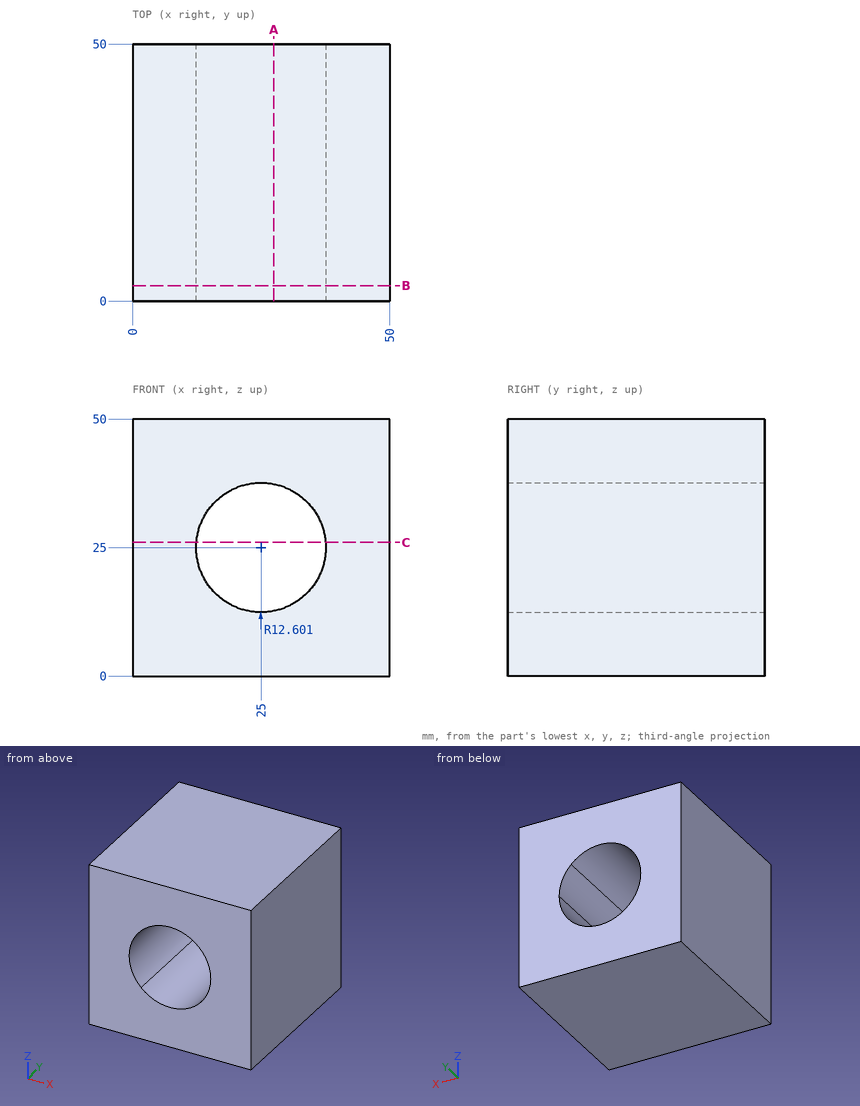
Print and shaded views of the part. All mm, measured from the part's lowest x, y and z. Round coordinates to 2 decimals unless told otherwise and drop trailing zeros. Write each loop counter-clockwise with the first axis right and the second up, starting at its lowest first coordinate (ties: lowest second). Pieces come first, ordered by that corner, then holes. Notation, with made-up numbers: (45.5, 68.5) -> (69.5, 68.5) arc R28 ccw to (69.5, 97.5) -> close; hole circle Ø1 at (28, -9.75). An arc over 180 degrees is marked (long way). Return JSON: item names as keys, results as strings. Group by question number.
Q1. Probe L1, parallel to Z at x = 30, y = 38 (1 decimal); L2, parallel to Z at x = 26, y = 14.5; L3, parallel to X at y = 19, z = 19.5. List the from-to ranges inside material, lowest first. Write a range as [from, to].
Q2. Saw through at B-B on y = 3. Write the cut outline in (x, z).
Q3. Saw through at C-C on z = 26. Write the cut outline in (x, y).
Q4. Saw through at A-A on x = 27.5. Write the cut outline in (y, z).
Answer:
{
 "1": {"L1": "[0, 13.4], [36.6, 50]", "L2": "[0, 12.44], [37.56, 50]", "L3": "[0, 13.66], [36.34, 50]"},
 "2": {"outline": "(0, 0) -> (50, 0) -> (50, 50) -> (0, 50) -> close; hole (16.09, 16.09) arc R12.6 ccw to (33.91, 16.09) arc R12.6 ccw to (37.6, 25) arc R12.6 ccw to (33.91, 33.91) arc R12.6 ccw to (16.09, 33.91) arc R12.6 ccw to start"},
 "3": {"outline": "(0, 0) -> (12.44, 0) -> (12.44, 50) -> (0, 50) -> close; (37.56, 0) -> (50, 0) -> (50, 50) -> (37.56, 50) -> close"},
 "4": {"outline": "(0, 0) -> (50, 0) -> (50, 12.65) -> (0, 12.65) -> close; (0, 37.35) -> (50, 37.35) -> (50, 50) -> (0, 50) -> close"}
}
